Autodesk Inventor part; units mm, degrees
ref_plane "YZ Plane" through (0, 0, 0) normal (1, 0, 0) x (0, 1, 0)
ref_plane "XZ Plane" through (0, 0, 0) normal (0, 1, 0) x (-1, 0, 0)
ref_plane "XY Plane" through (0, 0, 0) normal (0, 0, 1) x (1, 0, 0)
sketch "Sketch1" plane through (0, 0, 0) normal (0, 1, 0) x (-1, 0, 0)
  circle A0 centre (0, 0) radius 1.5
  dimension "d0" = 3
extrude "Extrusion1" add sketch "Sketch1" along normal blind 20
sketch "Sketch2" plane through (0, 20, 0) normal (0, 1, 0) x (1, 0, 0)
  circle A0 centre (0, 0) radius 2.5
  dimension "d3" = 5
extrude "Extrusion2" add sketch "Sketch2" along normal blind 2
fillet "Fillet1" radius 1.7 1 edges at (-2.5, 22, 0)
chamfer "Chamfer1" distance 0.3 angle 45 1 edges at (1.5, 0, 0)
thread "Thread1"
properties part number "M3x20 Screw Nylon" material "Nylon 6"
Input: part model. Units: mm. Frame: model coordinates. A direction names the side the tool comes from. Coordinates: 2 decimals unless noted, no trailing zeros. Write each loop counter-clockwise with the first axis right and the second up, starting at its lowest first coordinate (ties: lowest second). Pieces come first, ordered by that corner, then holes. Notation, with made-up numbers: (-19.75, 81) -> (3.25, 81) arc R28 ccw to (3.25, 120) -> close; hole circle Ø8 at (59.5, 1). An arc over 180 degrees is marked (long way). Answer as a JSON object with one key per item and string values.
1. Material intervals for line 1 (Z direction, x = 0.9, y = 2.5); line 2 (X direction, y = 6.5, z = -0.7); line 3 (Z direction, x = 1.55, y = 20.25), sorted ascending. Write a range as from..to.
Result set:
{"line 1": "z = -1.2..1.2", "line 2": "x = -1.33..1.33", "line 3": "z = -1.96..1.96"}
2. Mould query, pull axis Z, two halves, no side actions, for faces 1 (the face through (1.15, 20.15, -2.22)), 2 (the face through (0, 22, 0)). Classes: released by +Z, released by -Z, zero draft, split by the parting line, or undercut.
Result set:
{"face 1": "split by the parting line", "face 2": "zero draft"}
3. Section A-A on y = 16.5. Return the cut outline in (x, z).
Result set:
{"outline": "circle Ø3 at (0, 0)"}
4. Access query for faces 3 (the face through (0, 0, 0)), 4 (the face through (1.5, 10.01, -0.07)). Directions: +Z, -Z, +X, -X, +Y, -Y. A direction counts if a zero-diameter tool reaches every point of the face in a straight line with its end or side. Return the directions, or none.
Result set:
{"face 3": "+Z, -Z, +X, -X, -Y", "face 4": "-Y"}
5. First-contact query: P1, Ø1.5, axis at y = 15.5, z = 1.5, coming from the +X side; P2, Ø1.5, axis at x = 1, y = 13.5, coming from the -Z side; P3, Ø2, axis at y = 4, z = 0, coming from the +X side. Flat tips, straight axial feed; report the tip coordinate or a pass-through.
Result set:
{"P1": "stops at x = 1.3", "P2": "stops at z = -1.48", "P3": "stops at x = 1.5"}
